from build123d import *

# Parameters (mm, degrees)
BOSS_EXTRUDE1_DEPTH = 12
SHELL1_T            = -2
SKETCH3_R           = 2.75
CUT_EXTRUDE1_DEPTH  = 2
BOSS_EXTRUDE2_START = 10
SKETCH4_R           = 4.5
SKETCH4_R_2         = 2.75
BOSS_EXTRUDE2_DEPTH = 10
BOSS_EXTRUDE7_DEPTH = 10
SKETCH10_W          = 20
SKETCH10_H          = 40
CUT_EXTRUDE3_DEPTH  = 10
SKETCH9_R           = 3.45
SKETCH9_R_2         = 1
BOSS_EXTRUDE9_DEPTH = 18
CUT_EXTRUDE4_START  = -10
SKETCH11_R          = 1
CUT_EXTRUDE4_DEPTH  = 10


with BuildPart() as part:
    # Sketch1 → Boss-Extrude1 (new body)
    with BuildSketch(Plane(origin=(0, 0, 0), x_dir=(1, 0, 0), z_dir=(0, 1, 0))):
        with BuildLine():
            Line((-50, 20), (50, 20))
            ThreePointArc((50, 20), (70, 0), (50, -20))
            Line((50, -20), (-50, -20))
            ThreePointArc((-50, -20), (-70, 0), (-50, 20))
        make_face()
    extrude(amount=BOSS_EXTRUDE1_DEPTH)

    # Shell1
    shell1_openings = [part.faces().sort_by_distance(p)[0] for p in [
        (0, 12, 0),
    ]]
    offset(amount=SHELL1_T, openings=shell1_openings, kind=Kind.INTERSECTION)

    # Sketch3 → Cut-Extrude1 (cut)
    with BuildSketch(Plane(origin=(0, 2, 0), x_dir=(1, 0, 0), z_dir=(0, 1, 0))):
        with Locations(Location((-50, 0, 0), (0, 0, 270))):
            Circle(SKETCH3_R)
    extrude(amount=-CUT_EXTRUDE1_DEPTH, mode=Mode.SUBTRACT)

    # Sketch4 → Boss-Extrude2 (add)
    # profile 1 of 3: a face of its own
    with BuildSketch(Plane(origin=(0, 2, 0), x_dir=(1, 0, 0), z_dir=(0, 1, 0)).offset(BOSS_EXTRUDE2_START)):
        with Locations(Location((-50, 0, 0), (0, 0, 270))):
            Circle(SKETCH4_R)
        with Locations(Location((-50, 0, 0), (0, 0, 270))):
            Circle(SKETCH4_R_2, mode=Mode.SUBTRACT)
    # profile 2 of 3: a face of its own
    with BuildSketch(Plane(origin=(0, 2, 0), x_dir=(1, 0, 0), z_dir=(0, 1, 0)).offset(BOSS_EXTRUDE2_START)):
        with BuildLine():
            ThreePointArc((-47.25, 0), (-47.55434058, 1.257477634), (-48.4, 2.236626925))
            Line((-48.4, 2.236626925), (-48.4, -2.236626925))
            ThreePointArc((-48.4, -2.236626925), (-47.55434058, -1.257477634), (-47.25, 0))
        make_face()
    # profile 3 of 3: a face of its own
    with BuildSketch(Plane(origin=(0, 2, 0), x_dir=(1, 0, 0), z_dir=(0, 1, 0)).offset(BOSS_EXTRUDE2_START)):
        with BuildLine():
            Line((-51.6, -2.236626925), (-51.6, 2.236626925))
            ThreePointArc((-51.6, 2.236626925), (-52.75, 0), (-51.6, -2.236626925))
        make_face()
    extrude(amount=-BOSS_EXTRUDE2_DEPTH)

    # Sketch7 → Boss-Extrude7 (add)
    with BuildSketch(Plane(origin=(0, 2, 0), x_dir=(1, 0, 0), z_dir=(0, 1, 0))):
        with BuildLine():
            Line((-51, 17.972200756), (-51, 4.387482194))
            ThreePointArc((-51, 4.387482194), (-50, 4.5), (-49, 4.387482194))
            Line((-49, 4.387482194), (-49, 17.972200756))
            ThreePointArc((-49, 17.972200756), (-49.499806838, 17.993048847), (-50, 18))
            ThreePointArc((-50, 18), (-50.500193162, 17.993048847), (-51, 17.972200756))
        make_face()
        with BuildLine():
            Line((-51, 18), (-51, 17.972200756))
            ThreePointArc((-51, 17.972200756), (-50.500193162, 17.993048847), (-50, 18))
            Line((-50, 18), (-51, 18))
        make_face()
        with BuildLine():
            ThreePointArc((-50, 18), (-49.499806838, 17.993048847), (-49, 17.972200756))
            Line((-49, 17.972200756), (-49, 18))
            Line((-49, 18), (-50, 18))
        make_face()
        with BuildLine():
            Line((-32.027799244, 1), (-45.612517806, 1))
            ThreePointArc((-45.612517806, 1), (-45.528217924, 0.503155109), (-45.5, 0))
            ThreePointArc((-45.5, 0), (-45.528217924, -0.503155109), (-45.612517806, -1))
            Line((-45.612517806, -1), (-32.027799244, -1))
            ThreePointArc((-32.027799244, -1), (-32.006951153, -0.500193162), (-32, 0))
            ThreePointArc((-32, 0), (-32.006951153, 0.500193162), (-32.027799244, 1))
        make_face()
        with BuildLine():
            ThreePointArc((-49, -4.387482194), (-50, -4.5), (-51, -4.387482194))
            Line((-51, -4.387482194), (-51, -17.972200756))
            ThreePointArc((-51, -17.972200756), (-50.500193162, -17.993048847), (-50, -18))
            ThreePointArc((-50, -18), (-49.499806838, -17.993048847), (-49, -17.972200756))
            Line((-49, -17.972200756), (-49, -4.387482194))
        make_face()
        with BuildLine():
            Line((-49, -18), (-49, -17.972200756))
            ThreePointArc((-49, -17.972200756), (-49.499806838, -17.993048847), (-50, -18))
            Line((-50, -18), (-49, -18))
        make_face()
        with BuildLine():
            ThreePointArc((-54.387482194, -1), (-54.5, 0), (-54.387482194, 1))
            Line((-54.387482194, 1), (-67.972200756, 1))
            ThreePointArc((-67.972200756, 1), (-67.993048847, 0.500193146), (-68, -3.2e-08))
            ThreePointArc((-68, -3.2e-08), (-67.993048846, -0.500193178), (-67.972200756, -1))
            Line((-67.972200756, -1), (-54.387482194, -1))
        make_face()
    extrude(amount=BOSS_EXTRUDE7_DEPTH)

    # Sketch10 → Cut-Extrude3 (cut)
    with BuildSketch(Plane(origin=(0, 12, 0), x_dir=(1, 0, 0), z_dir=(0, 1, 0))):
        with Locations((60, 0)):
            Rectangle(SKETCH10_W, SKETCH10_H)
    extrude(amount=-CUT_EXTRUDE3_DEPTH, mode=Mode.SUBTRACT)

    # Sketch9 → Boss-Extrude9 (add)
    # profile 1 of 2: a face of its own
    with BuildSketch(Plane(origin=(0, 2, 0), x_dir=(1, 0, 0), z_dir=(0, 1, 0))):
        with Locations(Location((50, -17.5, 0), (0, 0, 188.333082996))):
            Circle(SKETCH9_R)
        with Locations(Location((50, -17.5, 0), (0, 0, 270))):
            Circle(SKETCH9_R_2, mode=Mode.SUBTRACT)
    # profile 2 of 2: a face of its own
    with BuildSketch(Plane(origin=(0, 2, 0), x_dir=(1, 0, 0), z_dir=(0, 1, 0))):
        with Locations(Location((50, 17.5, 0), (0, 0, 90))):
            Circle(SKETCH9_R)
        with Locations(Location((50, 17.5, 0), (0, 0, 90))):
            Circle(SKETCH9_R_2, mode=Mode.SUBTRACT)
    extrude(amount=BOSS_EXTRUDE9_DEPTH)

    # Sketch11 → Cut-Extrude4 (cut)
    with BuildSketch(Plane(origin=(0, 12, 0), x_dir=(1, 0, 0), z_dir=(0, 1, 0)).offset(CUT_EXTRUDE4_START)):
        with Locations(Location((50, 17.5, 0), (0, 0, 90))):
            Circle(SKETCH11_R)
        with Locations(Location((50, -17.5, 0), (0, 0, 270))):
            Circle(SKETCH11_R)
    extrude(amount=CUT_EXTRUDE4_DEPTH, mode=Mode.SUBTRACT)


solid = part.part
The model under review builds one solid part; all positions refer to its coordinate system, in mm. A direction names the side the tool comes from. Give positions to 0.01 mm unless a question says otherwise; leave off trailing zeros. Write each loop counter-clockwise with the first axis right and the second up, starting at its lowest first coordinate (ties: lowest second). Pieces come first, ordered by that corner, then holes. Notation, with made-up numbers: M 8.25,-2.75 L 38.25,-2.75 A13 cw 38.25,14.25 Z; hole C -3.5,88 d2. An arc over 180 degrees is marked long. One line per question, with ' | ' between items. Start each with the question number.
Item 1: We need section B-B on x = -43. Write out the cut boundary in (y, z).
Item 2: For faces 1 (the flat face through (50.92, 20, 18.19)), 2 (the flat face through (1, 0, 0)), 3 (the flat face through (-51.6, 7, 0)), 4 (the flat face through (-39, 7, 1)), 5 (the flat face through (-51, 7, 11)), list the 3-axis set-ups (+Z, -Z, +X, -X, +Y, -Y) from which the entire face can be reached by the end or side of a thin tool; tool diameter is ignored.
Item 3: Wall thickness on line 1 (Z direction, x = -6.5, y = 6.25); line 2 (X direction, y = 16.5, z = -17.5); line 3 (X direction, y = 3.5, z = 0): over which ranges is each line inside the solid? List them lowest first. Write a range as from..to.
Item 4: For pin 1 (6 mm diameter, centred on x = -9.5, y = 11, fed in from +Z); pin 2 (5 mm diameter, centred on x = -48.5, z = -12.5, fed in from +Y); pin 3 (20 mm diameter, centred on x = 17.5, z = -7, fed in from +Y); pin 4 (6 mm diameter, centred on y = 16.5, z = 8, fed in from +X), all flat-tipped, find the tip position at first contact; note any pin that passes through.
Item 5: We need section C-C on y = 6. Write out the cut boundary in (x, z), plus the area to 3 significant figures.
Item 6: Draft analysis for pull direction X (two halves, no side actions). For faces 6 (the flat face through (1, 6, 20)), 7 (the cylindrical face through (-46.793, 7.07, -3.157)), 8 (the flat face through (-2, 7, -18)), state which applies: released by +X, released by -X, zero draft, split by the parting line, or undercut.
Item 7: We need section A-A on y = 18. Write out the cut boundary in (x, z), plus the area to 3 significant figures.
Item 8: We need section D-D on z = 6. Write out the cut boundary in (x, y), plus the area to 3 significant figures.
Results found:
1) outline: M 0,-20 L 12,-20 L 12,-18 L 2,-18 L 2,-1 L 12,-1 L 12,1 L 2,1 L 2,18 L 12,18 L 12,20 L 0,20 Z
2) face 1: +Z, -Z, +X, -X, +Y | face 2: +Z, -Z, +X, -X, -Y | face 3: +Y, -Y | face 4: +X, +Y | face 5: +Y
3) line 1: z = -20..-18, 18..20 | line 2: x = 46.55..49, 51..53.45 | line 3: x = -70..-51.6, -48.4..-32
4) pin 1: stops at z = 20 | pin 2: stops at y = 12 | pin 3: stops at y = 2 | pin 4: passes through
5) outline: M -50,-20 L 47.62,-20 A3.45 ccw long 46.59,-18 L -49,-18 L -49,-4.39 A4.5 ccw -45.61,-1 L -32.03,-1 A18 ccw -32.03,1 L -45.61,1 A4.5 ccw -49,4.39 L -49,18 L 46.59,18 A3.45 ccw long 47.62,20 L -50,20 A20 ccw Z; hole M -67.97,-1 A18 ccw -51,-17.97 L -51,-4.39 A4.5 cw -54.39,-1 Z; hole M -67.97,1 L -54.39,1 A4.5 cw -51,4.39 L -51,17.97 A18 ccw Z; hole M -51.6,-2.24 A2.75 ccw -48.4,-2.24 L -48.4,2.24 A2.75 ccw -51.6,2.24 Z; hole C 50,-17.5 d2; hole C 50,17.5 d2 | area: 731 mm2
6) face 6: zero draft | face 7: released by +X | face 8: undercut
7) outline: C 50,-17.5 d6.9; C 50,17.5 d6.9; hole C 50,-17.5 d2; hole C 50,17.5 d2 | area: 68.5 mm2
8) outline: M -69.08,0 L 69.08,0 L 69.08,2 L -49,2 L -49,12 L -51,12 L -51,2 L -66.97,2 L -66.97,12 L -69.08,12 Z | area: 317 mm2
